Could you check a few things on this model? Use its own coordinates, in mm. A direction names the side the tool comes from. Coordinates: 2 decimals unless noted, no trailing zeros. Write each loop counter-clockwise with the first axis right and the second up, starting at its lowest first coordinate (ties: lowest second). Pieces come first, ordered by that corner, then holes.
```python
from build123d import *

# Parameters (mm, degrees)
F0_R     = 30.48
F1_DEPTH = 7.9375
F2_R     = 1.5
F3_DEPTH = 32.0605350826


# Not quite as in the source:
# - a length typed as a fraction of an inch, garbled in the dataset ("3 / 203.2 mm" for 3/8 in), is restored


with BuildPart() as f1:
    # F0 (on Top) → F1 (new body)
    with BuildSketch(Plane.XY):
        with BuildLine():
            Line((-64.135, -7.62), (-44.704, -33.528))
            ThreePointArc((-44.704, -33.528), (0, -55.88), (44.704, -33.528))
            Line((44.704, -33.528), (64.135, -7.62))
            ThreePointArc((64.135, -7.62), (66.675, 0), (64.135, 7.62))
            Line((64.135, 7.62), (44.704, 33.528))
            ThreePointArc((44.704, 33.528), (0, 55.88), (-44.704, 33.528))
            Line((-44.704, 33.528), (-64.135, 7.62))
            ThreePointArc((-64.135, 7.62), (-66.675, 0), (-64.135, -7.62))
        make_face()
        with BuildLine():
            ThreePointArc((-53.975, -6.477), (-60.452, 0), (-53.975, 6.477))
            Line((-53.975, 6.477), (-44.069, 6.477))
            ThreePointArc((-44.069, 6.477), (-37.592, 0), (-44.069, -6.477))
            Line((-44.069, -6.477), (-53.975, -6.477))
        make_face(mode=Mode.SUBTRACT)
        Circle(F0_R, mode=Mode.SUBTRACT)
        with BuildLine():
            ThreePointArc((44.069, -6.477), (37.592, 0), (44.069, 6.477))
            Line((44.069, 6.477), (53.9750001618, 6.477))
            ThreePointArc((53.9750001618, 6.477), (60.452, -8.09e-08), (53.975, -6.477))
            Line((53.975, -6.477), (44.069, -6.477))
        make_face(mode=Mode.SUBTRACT)
    extrude(amount=F1_DEPTH)

    # F2 (on face) → F3 (cut, up to face)
    with BuildSketch(Plane(origin=(-44.704, 33.528, 0), x_dir=(-0.6, -0.8, 0), z_dir=(-0.8, 0.6, 0))):
        with Locations((16.1925, 3.96875)):
            Circle(F2_R)
    extrude(amount=-F3_DEPTH, mode=Mode.SUBTRACT)


solid = f1.part
```
Item 1: Will these pins go through, and if not, where does the flat tip stop? pin 1 Ø1 at (y, z) = (16.5, 6.5) entering from +X; pin 2 Ø3 at (y, z) = (25, 2.5) entering from +X (3 decimals); pin 3 Ø4 at (x, z) = (47.5, 2.5) entering from +Y.
Item 2: Which directions (+Z, -Z, +X, -X, +Y, -Y) give clear straight access to the entire face, cutting with the end or side of a thin tool? Please do faces 1 (the flat face through (-49, -6.477, 4)), 2 (the flat face through (-31, 1, 0)).
Item 3: I want a section at A-A, the plane x = 0. List the corners of the cut face in (y, z) for me.
Item 4: I want a section at C-C, the plane y = 15.5. Count the separate pieces of the cut face and the enclosed holes in it, then the cut area to 3 significant figures.
Item 5: If I drill on line 1 along Y through (x, z) = (12.5, 7.25); line 2 along Y through (x, z) = (18, 7.75); line 3 along X through (y, z) = (25.5, 5.25) (3 decimals), over which ranges is the centre line in solid material (lowest first)?
Item 6: If we mould it in two halves opening along Y, with no side actions, what happens to faces 3 (the cylindrical face through (-0.725, -55.875, 3.913)), 4 (the flat face through (49, -6.477, 4)), 5 (the cylindrical face through (29.07, 9.16, 3.91)), 6 (the cylindrical face through (-66.674, 0.114, 3.913))? For each: released by +Y, released by -Y, zero draft, split by the parting line, or undercut.
Item 7: I want a section at B-B, the plane y = -14. List the corners of the cut face in (x, z) for me, then the cut area to 3 significant figures.
Taken from the geometry:
1. pin 1: stops at x = 57.85
1. pin 2: stops at x = 52.225
1. pin 3: stops at y = 32.47
2. face 1: +Z, -Z
2. face 2: -Z, +X, -X, +Y, -Y
3. outline: (-55.88, 0) - (-30.48, 0) - (-30.48, 7.94) - (-55.88, 7.94) - close; (30.48, 0) - (55.88, 0) - (55.88, 7.94) - (30.48, 7.94) - close
4. separate pieces: 2
4. enclosed holes: 1
4. area: 496 mm2
5. line 1: y = -54.46 to -27.8, 27.8 to 54.46
5. line 2: y = -52.9 to -24.6, 24.6 to 52.9
5. line 3: x = -50.725 to -16.697, 16.697 to 50.725
6. face 3: released by -Y
6. face 4: undercut
6. face 5: undercut
6. face 6: split by the parting line
7. outline: (-59.35, 0) - (-27.07, 0) - (-27.07, 7.94) - (-59.35, 7.94) - close; (27.07, 0) - (59.35, 0) - (59.35, 7.94) - (27.07, 7.94) - close
7. area: 512 mm2
